Job drawing, mm, ordinate dimensions from the low corner. One solid piece. A direction names the side the tool comes from. Coordinates: 2 decimals unless noted, no trailing zeros. Loops run counter-clockwise (first coordinate to the right, second up) from the corner with the lowest first, then second, coordinate; pieces in that order, holes last. Notation, with made-up numbers: (54.25, 35.5) - (65.25, 35.5) arc R11 cw to (65.25, 54.5) - close; hole circle Ø11 at (68.25, -6). An arc over 180 degrees is marked (long way). Use a Markdown table: item, result. Add a question column.
1. Drop flat-ended pins along their axis: pin 1 (10 mm diameter, centred on x = 48, z = 39, fed in from -Y); pin 2 (3.5 mm diameter, centred on y = 20, z = 1, fed in from -X); pin 3 (8 mm diameter, centred on y = 40.5, z = 39, fed in from +X); pin 4 (9.5 mm diameter, centred on x = 24, y = 17.5, fed in from +Z). Give the stop position or say it passes through.
2. 3-axis set-ups, long thin cutter, end or side, ignore diameter. For the marked faces 1 and 2: which of +Z, -Z, +X, -X, +Y, -Y reach the whole face in a straight line?
3. Band-saw the part on C-C, the plane y = 11. Give the cut face in (x, z) (1 decimal).
4. Band-saw the part on A-A, the plane x = 37. Give the cut face in (y, z).
5. Wall check: probe 1 along Z at (x, y) = (15.5, 37); probe 2 along Z at (x, y) = (50, 25.5); probe 3 along Y at (x, z) = (49, 36.5). Give the ranges that are in metal, low to high. Write a range as [from, to].
6. Band-saw the part on B-B, the plane y = 6. Give the cut face in (x, z) (1 decimal).
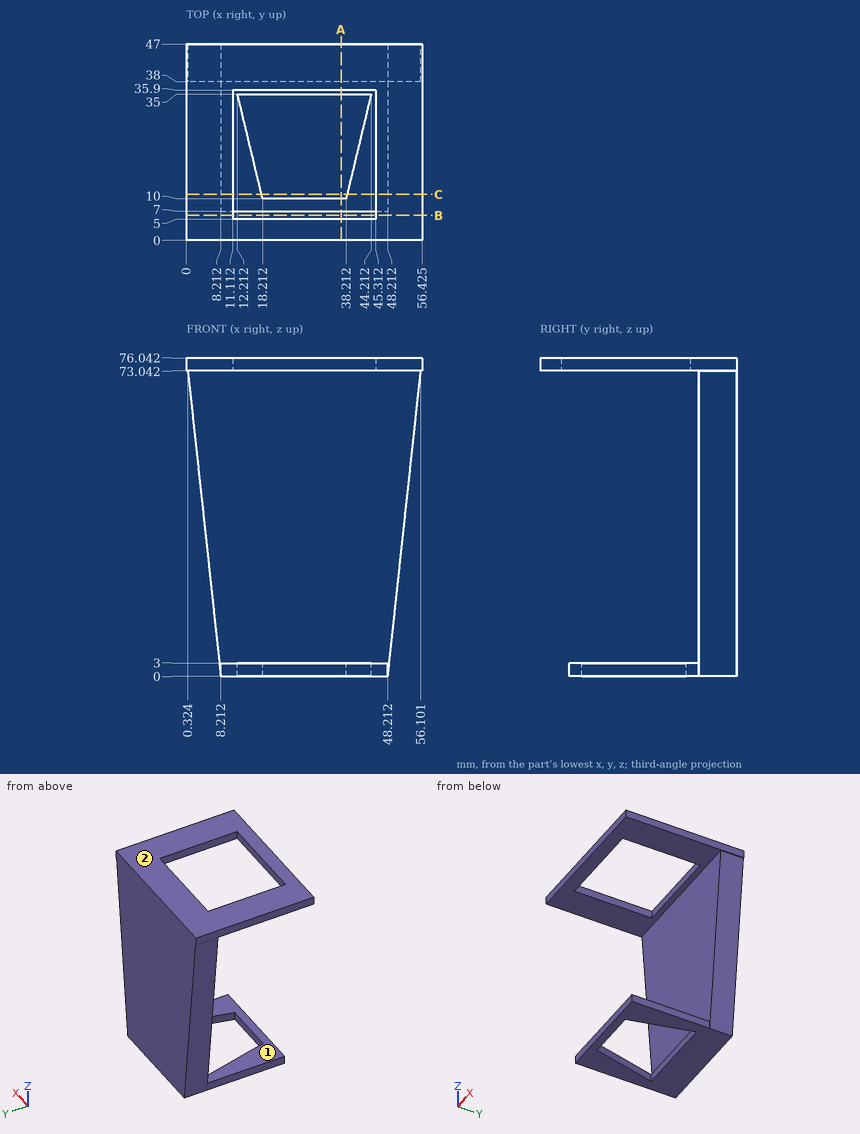
Geometry check:
| question | item | result |
|---|---|---|
| 1 | pin 1 | stops at y = 38 |
| 1 | pin 2 | stops at x = 8.21 |
| 1 | pin 3 | stops at x = 52.86 |
| 1 | pin 4 | passes through |
| 2 | face 1 | +X, -X, -Y |
| 2 | face 2 | +Z, +X, -X, +Y, -Y |
| 3 | outline | (0, 73) - (11.1, 73) - (11.1, 76) - (0, 76) - close; (8.2, 0) - (18, 0) - (18, 3) - (8.2, 3) - close; (38.5, 0) - (48.2, 0) - (48.2, 3) - (38.5, 3) - close; (45.3, 73) - (56.4, 73) - (56.4, 76) - (45.3, 76) - close |
| 4 | outline | (0, 73.04) - (5, 73.04) - (5, 76.04) - (0, 76.04) - close; (7, 0) - (10, 0) - (10, 3) - (7, 3) - close; (35, 0) - (47, 0) - (47, 76.04) - (35.9, 76.04) - (35.9, 73.04) - (38, 73.04) - (38, 3) - (35, 3) - close |
| 5 | probe 1 | z = [0, 3], [73.04, 76.04] |
| 5 | probe 2 | z = [73.04, 76.04] |
| 5 | probe 3 | y = [38, 47] |
| 6 | outline | (0, 73) - (11.1, 73) - (11.1, 76) - (0, 76) - close; (45.3, 73) - (56.4, 73) - (56.4, 76) - (45.3, 76) - close |
